```python
from build123d import *

# Parameters (mm, degrees)
SKETCH1_R           = 1.75
BOSS_EXTRUDE2_DEPTH = 3
SKETCH2_R           = 1.6
CUT_EXTRUDE1_DEPTH  = 3
FILLET1_R           = 4
SKETCH3_R           = 2
CUT_EXTRUDE2_DEPTH  = 3
SKETCH4_R           = 2
CUT_EXTRUDE3_DEPTH  = 3
SKETCH7_R           = 7.5
CUT_EXTRUDE5_DEPTH  = 3
SKETCH8_R           = 2
CUT_EXTRUDE7_DEPTH  = 3
SKETCH9_R           = 0.5
CUT_EXTRUDE8_DEPTH  = 3


with BuildPart() as part:
    # Sketch1 → Boss-Extrude2 (new body)
    with BuildSketch(Plane(origin=(0, 0, 0), x_dir=(1, 0, 0), z_dir=(0, 1, 0))):
        Polygon((-17.06639584, -5), (-8.5, -129.5), (-8.5, -134.5), (-8.5, -139.5), (92.5, -139.5), (92.5, -129.5), (101.06639584, -5), (101.06639584, 5), (96.06639584, 5), (-17.06639584, 5), (-17.06639584, 0), align=None)
        with Locations(Location((-12.06639584, 0, 0), (0, 0, 270))):
            Circle(SKETCH1_R, mode=Mode.SUBTRACT)
        with Locations(Location((96.06639584, 0, 0), (0, 0, 270))):
            Circle(SKETCH1_R, mode=Mode.SUBTRACT)
        with BuildLine():
            Line((-3.5, -132.75), (3.5, -132.75))
            ThreePointArc((3.5, -132.75), (5.25, -134.5), (3.5, -136.25))
            Line((3.5, -136.25), (-3.5, -136.25))
            ThreePointArc((-3.5, -136.25), (-5.25, -134.5), (-3.5, -132.75))
        make_face(mode=Mode.SUBTRACT)
        with BuildLine():
            Line((87.5, -132.75), (80.5, -132.75))
            ThreePointArc((80.5, -132.75), (78.75, -134.5), (80.5, -136.25))
            Line((80.5, -136.25), (87.5, -136.25))
            ThreePointArc((87.5, -136.25), (89.25, -134.5), (87.5, -132.75))
        make_face(mode=Mode.SUBTRACT)
    extrude(amount=BOSS_EXTRUDE2_DEPTH)

    # Sketch2 → Cut-Extrude1 (cut)
    with BuildSketch(Plane(origin=(0, 3, 0), x_dir=(1, 0, 0), z_dir=(0, 1, 0))):
        with Locations(Location((11, -41.028359395, 0), (0, 0, 270))):
            Circle(SKETCH2_R)
        with Locations(Location((73, -41.028359395, 0), (0, 0, 270))):
            Circle(SKETCH2_R)
        with Locations(Location((17, -98.028359395, 0), (0, 0, 270))):
            Circle(SKETCH2_R)
        with Locations(Location((67, -98.028359395, 0), (0, 0, 270))):
            Circle(SKETCH2_R)
    extrude(amount=-CUT_EXTRUDE1_DEPTH, mode=Mode.SUBTRACT)

    # Fillet1
    fillet1_edges = [part.edges().sort_by_distance(p)[0] for p in [
        (-17.06639584, 1.5, -5),
        (101.06639584, 1.5, -5),
        (92.5, 1.5, 139.5),
        (-8.5, 1.5, 139.5),
    ]]
    fillet(fillet1_edges, radius=FILLET1_R)

    # Sketch3 → Cut-Extrude2 (cut)
    with BuildSketch(Plane(origin=(0, 3, 0), x_dir=(1, 0, 0), z_dir=(0, 1, 0))):
        with Locations(Location((42, 0, 0), (0, 0, 270))):
            Circle(SKETCH3_R)
        with Locations(Location((-3.5, -95, 0), (0, 0, 270))):
            Circle(SKETCH3_R)
        with Locations(Location((-3.5, -111, 0), (0, 0, 270))):
            Circle(SKETCH3_R)
        with Locations(Location((42, -134.5, 0), (0, 0, 270))):
            Circle(SKETCH3_R)
        with Locations(Location((-3.5, -122.75, 0), (0, 0, 270))):
            Circle(SKETCH3_R)
        with Locations(Location((12, -111, 0), (0, 0, 270))):
            Circle(SKETCH3_R)
        with Locations(Location((22, -111, 0), (0, 0, 270))):
            Circle(SKETCH3_R)
        with Locations(Location((32, -111, 0), (0, 0, 270))):
            Circle(SKETCH3_R)
        with Locations(Location((42, -111, 0), (0, 0, 270))):
            Circle(SKETCH3_R)
        with Locations(Location((52, -111, 0), (0, 0, 90))):
            Circle(SKETCH3_R)
        with Locations(Location((62, -111, 0), (0, 0, 90))):
            Circle(SKETCH3_R)
        with Locations(Location((72, -111, 0), (0, 0, 90))):
            Circle(SKETCH3_R)
        with Locations(Location((87.5, -122.75, 0), (0, 0, 90))):
            Circle(SKETCH3_R)
        with Locations(Location((87.5, -111, 0), (0, 0, 90))):
            Circle(SKETCH3_R)
        with Locations(Location((87.5, -95, 0), (0, 0, 90))):
            Circle(SKETCH3_R)
        with BuildLine():
            Line((23.519670138, -1.5), (3.519670138, -1.5))
            ThreePointArc((3.519670138, -1.5), (2.019670138, 0), (3.519670138, 1.5))
            Line((3.519670138, 1.5), (23.519670138, 1.5))
            ThreePointArc((23.519670138, 1.5), (25.019670138, 0), (23.519670138, -1.5))
        make_face()
        with BuildLine():
            Line((29.602369227, -136), (14.602369227, -136))
            ThreePointArc((14.602369227, -136), (13.102369227, -134.5), (14.602369227, -133))
            Line((14.602369227, -133), (29.602369227, -133))
            ThreePointArc((29.602369227, -133), (31.102369227, -134.5), (29.602369227, -136))
        make_face()
        with BuildLine():
            Line((54.397630773, -136), (69.397630773, -136))
            ThreePointArc((69.397630773, -136), (70.897630773, -134.5), (69.397630773, -133))
            Line((69.397630773, -133), (54.397630773, -133))
            ThreePointArc((54.397630773, -133), (52.897630773, -134.5), (54.397630773, -136))
        make_face()
        with BuildLine():
            Line((60.480329862, -1.5), (80.480329862, -1.5))
            ThreePointArc((80.480329862, -1.5), (81.980329862, 0), (80.480329862, 1.5))
            Line((80.480329862, 1.5), (60.480329862, 1.5))
            ThreePointArc((60.480329862, 1.5), (58.980329862, 0), (60.480329862, -1.5))
        make_face()
    extrude(amount=-CUT_EXTRUDE2_DEPTH, mode=Mode.SUBTRACT)

    # Sketch4 → Cut-Extrude3 (cut)
    with BuildSketch(Plane(origin=(0, 3, 0), x_dir=(1, 0, 0), z_dir=(0, 1, 0))):
        with Locations(Location((12, -122.75, 0), (0, 0, 270))):
            Circle(SKETCH4_R)
        with Locations(Location((22, -122.75, 0), (0, 0, 270))):
            Circle(SKETCH4_R)
        with Locations(Location((32, -122.75, 0), (0, 0, 270))):
            Circle(SKETCH4_R)
        with Locations(Location((42, -122.75, 0), (0, 0, 270))):
            Circle(SKETCH4_R)
        with Locations(Location((52, -122.75, 0), (0, 0, 270))):
            Circle(SKETCH4_R)
        with Locations(Location((62, -122.75, 0), (0, 0, 270))):
            Circle(SKETCH4_R)
        with Locations(Location((72, -122.75, 0), (0, 0, 270))):
            Circle(SKETCH4_R)
    extrude(amount=-CUT_EXTRUDE3_DEPTH, mode=Mode.SUBTRACT)

    # Sketch7 → Cut-Extrude5 (cut)
    with BuildSketch(Plane(origin=(0, 3, 0), x_dir=(1, 0, 0), z_dir=(0, 1, 0))):
        with Locations(Location((42, -69.75, 0), (0, 0, 270))):
            Circle(SKETCH7_R)
    extrude(amount=-CUT_EXTRUDE5_DEPTH, mode=Mode.SUBTRACT)

    # Sketch8 → Cut-Extrude7 (cut)
    with BuildSketch(Plane(origin=(0, 3, 0), x_dir=(1, 0, 0), z_dir=(0, 1, 0))):
        with Locations(Location((-3.5, -26.25, 0), (0, 0, 270))):
            Circle(SKETCH8_R)
        with Locations(Location((-3.5, -37, 0), (0, 0, 270))):
            Circle(SKETCH8_R)
        with Locations(Location((-3.5, -70.5, 0), (0, 0, 270))):
            Circle(SKETCH8_R)
        with Locations(Location((-3.5, -82.5, 0), (0, 0, 270))):
            Circle(SKETCH8_R)
        with Locations(Location((-3.5, -6.5, 0), (0, 0, 270))):
            Circle(SKETCH8_R)
        with Locations(Location((-3.5, -15.5, 0), (0, 0, 270))):
            Circle(SKETCH8_R)
        with Locations(Location((-3.5, -47.75, 0), (0, 0, 270))):
            Circle(SKETCH8_R)
        with Locations(Location((-3.5, -58.5, 0), (0, 0, 270))):
            Circle(SKETCH8_R)
        with Locations(Location((87.5, -6.5, 0), (0, 0, 90))):
            Circle(SKETCH8_R)
        with Locations(Location((87.5, -15.5, 0), (0, 0, 90))):
            Circle(SKETCH8_R)
        with Locations(Location((87.5, -26.25, 0), (0, 0, 90))):
            Circle(SKETCH8_R)
        with Locations(Location((87.5, -37, 0), (0, 0, 90))):
            Circle(SKETCH8_R)
        with Locations(Location((87.5, -47.75, 0), (0, 0, 90))):
            Circle(SKETCH8_R)
        with Locations(Location((87.5, -58.5, 0), (0, 0, 90))):
            Circle(SKETCH8_R)
        with Locations(Location((87.5, -70.5, 0), (0, 0, 90))):
            Circle(SKETCH8_R)
        with Locations(Location((87.5, -82.5, 0), (0, 0, 90))):
            Circle(SKETCH8_R)
    extrude(amount=-CUT_EXTRUDE7_DEPTH, mode=Mode.SUBTRACT)

    # Sketch9 → Cut-Extrude8 (cut)
    with BuildSketch(Plane(origin=(0, 3, 0), x_dir=(1, 0, 0), z_dir=(0, 1, 0))):
        with Locations(Location((42, -19.310550248, 0), (0, 0, 270))):
            Circle(SKETCH9_R)
    extrude(amount=-CUT_EXTRUDE8_DEPTH, mode=Mode.SUBTRACT)


solid = part.part
```
Design review of the part built by this model. Coordinates are the model's own, in mm. A direction names the side the tool comes from. Coordinates: 2 decimals unless noted, no trailing zeros. Loops run counter-clockwise (first coordinate to the right, second up) from the corner with the lowest first, then second, coordinate; pieces in that order, holes last. Notation, with made-up numbers: (77.5, -25.75) -> (89.5, -25.75) arc R18 cw to (89.5, 9.25) -> close; hole circle Ø1 at (50, 73). An arc over 180 degrees is marked (long way). Answer as a JSON object with one key per item and string values.
Q1. The part is to be moulded in two halves that separate along X. For faces 1 (the flat face through (101.066, 1, 2)), 2 (the cylindrical face through (40.8, 1.5, 132.9)), 3 (the flat face through (-17.066, 1, 2)), say which applies: +X half, -X half, draft (parallel to the pull), parting line (faces both ways), or undercut.
Answer block:
{"face 1": "+X half", "face 2": "undercut", "face 3": "-X half"}
Q2. Take a section at C-C on z = 26.25. Give the boundary of the cut face in (x, y), plus the area to 3 significant figures.
Answer block:
{"outline": "(-15.6, 0) -> (-5.5, 0) -> (-5.5, 3) -> (-15.6, 3) -> close; (-1.5, 0) -> (85.5, 0) -> (85.5, 3) -> (-1.5, 3) -> close; (89.5, 0) -> (99.6, 0) -> (99.6, 3) -> (89.5, 3) -> close", "area": "322 mm^2"}
Q3. Tool access review of faces 4 (the flat face through (0, 1, 132.75)), 5 (the cylindrical face through (99.864, 1.521, -3.859)): name each direction out of +Z, -Z, +X, -X, +Y, -Y from which nothing blocks a thin tool from reaching the whole face with its end or side.
Answer block:
{"face 4": "+Y, -Y", "face 5": "-Z, +X, +Y, -Y"}
Q4. Clearance check with a flat-ended pin moving along its axis: pin 1 Ø2.5 at (x, z) = (-3.5, 58.5) entering from -Y. State where the tip first meets the part, or that it passes through.
Answer block:
{"pin 1": "passes through"}
Q5. Take a section at D-D on z = 70.5. Give the boundary of the cut face in (x, y).
Answer block:
{"outline": "(-12.56, 0) -> (-5.5, 0) -> (-5.5, 3) -> (-12.56, 3) -> close; (-1.5, 0) -> (34.54, 0) -> (34.54, 3) -> (-1.5, 3) -> close; (49.46, 0) -> (85.5, 0) -> (85.5, 3) -> (49.46, 3) -> close; (89.5, 0) -> (96.56, 0) -> (96.56, 3) -> (89.5, 3) -> close"}
Q6. Take a section at A-A on x = 27. Give the boundary of the cut face in (y, z).
Answer block:
{"outline": "(0, -5) -> (3, -5) -> (3, 133) -> (0, 133) -> close; (0, 136) -> (3, 136) -> (3, 139.5) -> (0, 139.5) -> close"}
Q7. To check wall thickness, follow L1, parallel to Z at x = 67, y = 0.4; L2, parallel to Z at x = -1, y = 2.45; L3, parallel to X at y = 1.8, z = 0. State the ranges of each line that lie inside material, in increasing order.
Answer block:
{"L1": "z = -5 to -1.5, 1.5 to 96.43, 99.63 to 133, 136 to 139.5", "L2": "z = -5 to 132.75, 136.25 to 139.5", "L3": "x = -17.07 to -13.82, -10.32 to 2.02, 25.02 to 40, 44 to 58.98, 81.98 to 94.32, 97.82 to 101.07"}
Q8. Take a section at B-B on x = 67. Give the boundary of the cut face in (y, z).
Answer block:
{"outline": "(0, -5) -> (3, -5) -> (3, -1.5) -> (0, -1.5) -> close; (0, 1.5) -> (3, 1.5) -> (3, 96.43) -> (0, 96.43) -> close; (0, 99.63) -> (3, 99.63) -> (3, 133) -> (0, 133) -> close; (0, 136) -> (3, 136) -> (3, 139.5) -> (0, 139.5) -> close"}
